Geometry: final body of the model. Coordinates: model frame, mm. Coordinates: 2 decimals unless noted, no trailing zeros. Loops run counter-clockwise (first coordinate to the right, second up) from the corner with the lowest first, then second, coordinate; pieces in that order, holes last. Notation, with made-up numbers: (-5.5, 32.25) - (12.5, 32.25) arc R33 cw to (12.5, 65.25) - close; hole circle Ø3 at (76, 13). An arc over 180 degrees is marked (long way). Put each result on its own line as item: value. Start each with the question number.
1) Material intervals for line 1 along Y through (x, z) = (257, 0.4); line 2 along Y through (x, z) = (217, -1.4); line 3 along X through (y, z) = (93, 0.8), sorted ascending. Write a range as from..to.
2) Section A-A on y = 108.5. Output: boundary loops of the cut face in (x, z), and give its area (3 significant figures).
3) Section D-D on x = 197. Output: boundary loops of the cut face in (y, z).
4) Section B-B on y = 123.5. Output: boundary loops of the cut face in (x, z), and give its area (3 significant figures).
5) Section C-C on y = 50. Output: boundary loops of the cut face in (x, z), and give its area (3 significant figures).
6) Contact query for flat-ended pins moving along their axis: pin 1 Ø0.9 at (y, z) = (124.5, -0.5) entering from +X; pin 2 Ø0.9 at (y, z) = (64.5, 0.5) entering from +X; pin 3 Ø0.9 at (x, z) = (262, 0.5) entering from +Y. Output: stop coordinate, or through.
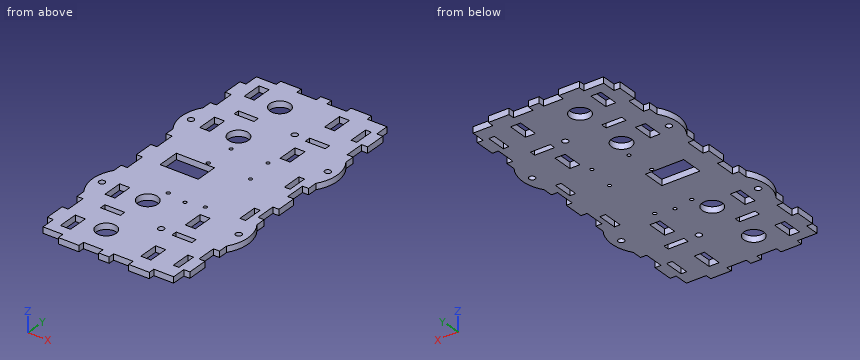
```python
from build123d import *

# Parameters (mm, degrees)
CROQUIS1_R                               = 1.5
CROQUIS1_R_2                             = 1.506117052
SALIENTE_EXTRUIR1_DEPTH                  = 1.5
CROQUIS3_W                               = 13
CROQUIS3_H                               = 10.999999999
CORTAR_EXTRUIR2_DEPTH                    = 10
TALADRO_DE_MARGEN_PARA_M1_61_D           = 1.7
TALADRO_DE_MARGEN_PARA_M1_61_CSINK_D     = 1.75
TALADRO_DE_MARGEN_PARA_M1_61_CSINK_ANGLE = 90
CROQUIS10_W                              = 5
CROQUIS10_H                              = 10
CORTAR_EXTRUIR3_DEPTH                    = 10
TALADRO_DE_MARGEN_PARA_M1_62_D           = 1.7
TALADRO_DE_MARGEN_PARA_M1_62_DEPTH       = 10
TALADRO_DE_MARGEN_PARA_M1_62_TIP         = 0.510731526
CROQUIS14_W                              = 2.8
CROQUIS14_H                              = 9.8
CORTAR_EXTRUIR4_DEPTH                    = 10
CROQUIS15_R                              = 5
CORTAR_EXTRUIR5_DEPTH                    = 10


with BuildPart() as part:
    # Croquis1 → Saliente-Extruir1 (new, symmetric)
    with BuildSketch(Plane.XY):
        with BuildLine():
            Line((205.355115241, 182.028523427), (195.480115242, 182.028523427))
            Line((195.480115242, 182.028523427), (195.480115242, 175.028523428))
            Line((195.480115242, 175.028523428), (192.480115242, 175.028523428))
            Line((192.480115242, 175.028523428), (192.480115242, 165.028523428))
            Line((192.480115242, 165.028523428), (195.480115242, 165.028523428))
            Line((195.480115242, 165.028523428), (195.480115242, 155.028523429))
            Line((195.480115242, 155.028523429), (192.480115242, 155.028523429))
            Line((192.480115242, 155.028523429), (192.480115242, 150.148106778))
            ThreePointArc((192.480115242, 150.148106778), (189.350724152, 139.96602343), (192.480115242, 129.783940083))
            Line((192.480115242, 129.783940083), (192.480115242, 125.153523431))
            Line((192.480115242, 125.153523431), (195.480115242, 125.153523431))
            Line((195.480115242, 125.153523431), (195.480115242, 114.903523432))
            Line((195.480115242, 114.903523432), (192.480115242, 114.903523432))
            Line((192.480115242, 114.903523432), (192.480115242, 105.153523433))
            Line((192.480115242, 105.153523433), (195.480115242, 105.153523433))
            Line((195.480115242, 105.153523433), (195.480115242, 94.903523434))
            Line((195.480115242, 94.903523434), (192.480115242, 94.903523434))
            Line((192.480115242, 94.903523434), (192.480115242, 90.023106782))
            ThreePointArc((192.480115242, 90.023106782), (189.350724152, 79.841023435), (192.480115242, 69.658940087))
            Line((192.480115242, 69.658940087), (192.480115242, 65.028523436))
            Line((192.480115242, 65.028523436), (195.480115242, 65.028523436))
            Line((195.480115242, 65.028523436), (195.480115242, 55.028523436))
            Line((195.480115242, 55.028523436), (192.480115242, 55.028523436))
            Line((192.480115242, 55.028523436), (192.480115242, 45.028523437))
            Line((192.480115242, 45.028523437), (195.480115242, 45.028523437))
            Line((195.480115242, 45.028523437), (195.480115242, 38.028637727))
            Line((195.480115242, 38.028637727), (205.355115241, 38.028637727))
            Line((205.355115241, 38.028637727), (205.355115241, 35.028637727))
            Line((205.355115241, 35.028637727), (215.605115241, 35.028637727))
            Line((215.605115241, 35.028637727), (215.605115241, 38.028620144))
            Line((215.605115241, 38.028620144), (225.355044383, 38.028620144))
            Line((225.355044383, 38.028620144), (225.355044383, 35.028598165))
            Line((225.355044383, 35.028598165), (230.605044383, 35.028598165))
            Line((230.605044383, 35.028598165), (230.605044383, 38.028598165))
            Line((230.605044383, 38.028598165), (240.354973525, 38.028598165))
            Line((240.354973525, 38.028598165), (240.354973525, 35.028589374))
            Line((240.354973525, 35.028589374), (250.604973524, 35.028589374))
            Line((250.604973524, 35.028589374), (250.604973524, 38.028580582))
            Line((250.604973524, 38.028580582), (260.479973524, 38.028580582))
            Line((260.479973524, 38.028580582), (260.479973524, 44.903580582))
            Line((260.479973524, 44.903580582), (263.479973523, 44.903580582))
            Line((263.479973523, 44.903580582), (263.479973523, 55.153580581))
            Line((263.479973523, 55.153580581), (260.479973524, 55.153580581))
            Line((260.479973524, 55.153580581), (260.479973524, 64.90358058))
            Line((260.479973524, 64.90358058), (263.479973523, 64.90358058))
            Line((263.479973523, 64.90358058), (263.479973523, 69.783997232))
            ThreePointArc((263.479973523, 69.783997232), (266.609364614, 79.966080579), (263.479973523, 90.148163927))
            Line((263.479973523, 90.148163927), (263.479973523, 95.028580578))
            Line((263.479973523, 95.028580578), (260.479973524, 95.028580578))
            Line((260.479973524, 95.028580578), (260.479973524, 105.028580577))
            Line((260.479973524, 105.028580577), (263.479973523, 105.028580577))
            Line((263.479973523, 105.028580577), (263.479973523, 115.028580577))
            Line((263.479973523, 115.028580577), (260.479973524, 115.028580577))
            Line((260.479973524, 115.028580577), (260.479973524, 125.028580576))
            Line((260.479973524, 125.028580576), (263.479973523, 125.028580576))
            Line((263.479973523, 125.028580576), (263.479973523, 129.908997227))
            ThreePointArc((263.479973523, 129.908997227), (266.609364614, 140.091080575), (263.479973523, 150.273163922))
            Line((263.479973523, 150.273163922), (263.479973523, 155.153580574))
            Line((263.479973523, 155.153580574), (260.479973524, 155.153580574))
            Line((260.479973524, 155.153580574), (260.479973524, 164.903580573))
            Line((260.479973524, 164.903580573), (263.479973523, 164.903580573))
            Line((263.479973523, 164.903580573), (263.479973523, 175.153580572))
            Line((263.479973523, 175.153580572), (260.479973524, 175.153580572))
            Line((260.479973524, 175.153580572), (260.479973524, 182.028580572))
            Line((260.479973524, 182.028580572), (250.604973524, 182.028580572))
            Line((250.604973524, 182.028580572), (250.604973524, 185.02857178))
            Line((250.604973524, 185.02857178), (240.354973525, 185.02857178))
            Line((240.354973525, 185.02857178), (240.354973525, 182.028562989))
            Line((240.354973525, 182.028562989), (230.605044383, 182.028562989))
            Line((230.605044383, 182.028562989), (230.605044383, 185.028562989))
            Line((230.605044383, 185.028562989), (225.355044383, 185.028562989))
            Line((225.355044383, 185.028562989), (225.355044383, 182.02854101))
            Line((225.355044383, 182.02854101), (215.605115241, 182.02854101))
            Line((215.605115241, 182.02854101), (215.605115241, 185.028523427))
            Line((215.605115241, 185.028523427), (205.355115241, 185.028523427))
            Line((205.355115241, 185.028523427), (205.355115241, 182.028523427))
        make_face()
        Polygon((215.180079812, 63.578494864), (210.095175212, 63.578494864), (205.280079813, 63.578494864), (205.280079813, 65.17614563), (205.280079813, 66.478494863), (210.095175212, 66.478494863), (215.180079812, 66.478494863), (215.180079812, 65.17614563), align=None, mode=Mode.SUBTRACT)
        with Locations((193.980115242, 79.841023435)):
            Circle(CROQUIS1_R, mode=Mode.SUBTRACT)
        Polygon((204.687627513, 115.528523432), (207.487627511, 115.528523432), (210.687627512, 115.528523432), (210.687627512, 109.828523436), (210.687627512, 104.528523433), (207.487627511, 104.528523433), (204.687627513, 104.528523433), (204.687627513, 110.228523436), align=None, mode=Mode.SUBTRACT)
        with Locations((234.380026668, 65.028523436)):
            Circle(CROQUIS1_R_2, mode=Mode.SUBTRACT)
        Polygon((250.680008953, 63.578523436), (245.595104353, 63.578523436), (240.780008954, 63.578523436), (240.780008954, 65.176174202), (240.780008954, 66.478523436), (245.595104353, 66.478523436), (250.680008953, 66.478523436), (250.680008953, 65.176174202), align=None, mode=Mode.SUBTRACT)
        with Locations((261.979973524, 79.966080579)):
            Circle(CROQUIS1_R, mode=Mode.SUBTRACT)
        with Locations((193.980115242, 139.96602343)):
            Circle(CROQUIS1_R, mode=Mode.SUBTRACT)
        Polygon((215.180079812, 153.675173656), (210.095175212, 153.675173656), (205.280079813, 153.675173656), (205.280079813, 155.272824422), (205.280079813, 156.575173656), (210.095175212, 156.575173656), (215.180079812, 156.575173656), (215.180079812, 155.272824422), align=None, mode=Mode.SUBTRACT)
        with Locations((261.979973524, 140.091080575)):
            Circle(CROQUIS1_R, mode=Mode.SUBTRACT)
        with Locations((234.380026668, 155.125202228)):
            Circle(CROQUIS1_R, mode=Mode.SUBTRACT)
        Polygon((250.680008953, 153.675202228), (245.864913553, 153.675202228), (240.780008954, 153.675202228), (240.780008954, 155.272852994), (240.780008954, 156.575202228), (245.864913553, 156.575202228), (250.680008953, 156.575202228), (250.680008953, 155.272852994), align=None, mode=Mode.SUBTRACT)
    extrude(amount=SALIENTE_EXTRUIR1_DEPTH, both=True)

    # Croquis3 → Cortar-Extruir2 (cut)
    with BuildSketch(Plane(origin=(0, 0, -1.5), x_dir=(-1, 0, 0), z_dir=(0, 0, -1))):
        with Locations((-217.187627512, 110.028523433)):
            Rectangle(CROQUIS3_W, CROQUIS3_H)
    extrude(amount=-CORTAR_EXTRUIR2_DEPTH, mode=Mode.SUBTRACT)

    # Taladro de margen para M1.61 (through all)
    with Locations(Plane(origin=(0, 0, -1.5), x_dir=(-1, 0, 0), z_dir=(0, 0, -1))):
        with Locations((-238.760115242, 131.208523432), (-220.340115242, 131.208523432), (-220.340115242, 88.848637722), (-238.760115242, 88.848637722)):
            CounterSinkHole(TALADRO_DE_MARGEN_PARA_M1_61_D / 2, TALADRO_DE_MARGEN_PARA_M1_61_CSINK_D / 2, counter_sink_angle=TALADRO_DE_MARGEN_PARA_M1_61_CSINK_ANGLE)

    # Croquis10 → Cortar-Extruir3 (cut)
    with BuildSketch(Plane(origin=(0, 0, -1.5), x_dir=(-1, 0, 0), z_dir=(0, 0, -1))):
        with Locations((-202.980115242, 142.028580577)):
            Rectangle(CROQUIS10_W, CROQUIS10_H)
        with Locations((-202.980115242, 172.028580577)):
            Rectangle(CROQUIS10_W, CROQUIS10_H)
        with Locations((-202.980115242, 78.028580577)):
            Rectangle(CROQUIS10_W, CROQUIS10_H)
        with Locations((-202.980115242, 48.028580577)):
            Rectangle(CROQUIS10_W, CROQUIS10_H)
        with Locations((-242.980115242, 48.028580577)):
            Rectangle(CROQUIS10_W, CROQUIS10_H)
        with Locations((-242.980115242, 78.028580577)):
            Rectangle(CROQUIS10_W, CROQUIS10_H)
        with Locations((-242.980115242, 172.028580577)):
            Rectangle(CROQUIS10_W, CROQUIS10_H)
        with Locations((-242.980115242, 142.028580577)):
            Rectangle(CROQUIS10_W, CROQUIS10_H)
    extrude(amount=-CORTAR_EXTRUIR3_DEPTH, mode=Mode.SUBTRACT)

    # Taladro de margen para M1.62
    with Locations(Plane(origin=(0, 0, -1.5), x_dir=(-1, 0, 0), z_dir=(0, 0, -1))):
        with Locations((-240.479973524, 117.029100767), (-219.479973524, 117.029100767), (-229.979973524, 87.029100767), (-170.093156085, 124.870857212)):
            Hole(TALADRO_DE_MARGEN_PARA_M1_62_D / 2, depth=TALADRO_DE_MARGEN_PARA_M1_62_DEPTH)
            with Locations((0, 0, -(TALADRO_DE_MARGEN_PARA_M1_62_DEPTH + TALADRO_DE_MARGEN_PARA_M1_62_TIP / 2))):  # 118° drill point
                Cone(0, TALADRO_DE_MARGEN_PARA_M1_62_D / 2, TALADRO_DE_MARGEN_PARA_M1_62_TIP, mode=Mode.SUBTRACT)

    # Croquis14 → Cortar-Extruir4 (cut)
    with BuildSketch(Plane(origin=(0, 0, -1.5), x_dir=(-1, 0, 0), z_dir=(0, 0, -1))):
        with Locations((-256.479973523, 170.028574939)):
            Rectangle(CROQUIS14_W, CROQUIS14_H)
        with Locations((-256.479973523, 50.028586215)):
            Rectangle(CROQUIS14_W, CROQUIS14_H)
        with Locations((-256.479973523, 95.028580577)):
            Rectangle(CROQUIS14_W, CROQUIS14_H)
        with Locations((-256.479973523, 125.028580577)):
            Rectangle(CROQUIS14_W, CROQUIS14_H)
    extrude(amount=-CORTAR_EXTRUIR4_DEPTH, mode=Mode.SUBTRACT)

    # Croquis15 → Cortar-Extruir5 (cut)
    with BuildSketch(Plane(origin=(0, 0, -1.5), x_dir=(-1, 0, 0), z_dir=(0, 0, -1))):
        with Locations((-217.080079819, 51.410663554)):
            Circle(CROQUIS15_R)
        with Locations((-217.080079819, 79.410663554)):
            Circle(CROQUIS15_R)
        with Locations(Location((-217.080079819, 140.6464976, 0), (0, 0, 180))):
            Circle(CROQUIS15_R)
        with Locations(Location((-217.080079819, 168.6464976, 0), (0, 0, 180))):
            Circle(CROQUIS15_R)
    extrude(amount=-CORTAR_EXTRUIR5_DEPTH, mode=Mode.SUBTRACT)


solid = part.part
```
Answer block:
1. line 1: y = 38.03..45.13, 54.93..90.13, 99.93..120.13, 129.93..165.13, 174.93..182.03
1. line 2: y = 38.03..46.41, 56.41..74.41, 84.41..104.53, 115.53..135.65, 145.65..163.65, 173.65..182.03
1. line 3: x = 192.48..255.08, 257.88..263.48
2. outline: (192.48, -1.5) - (204.69, -1.5) - (204.69, 1.5) - (192.48, 1.5) - close; (223.69, -1.5) - (263.48, -1.5) - (263.48, 1.5) - (223.69, 1.5) - close
2. area: 156 mm²
3. outline: (38.03, -1.5) - (182.03, -1.5) - (182.03, 1.5) - (38.03, 1.5) - close
4. outline: (195.48, -1.5) - (255.08, -1.5) - (255.08, 1.5) - (195.48, 1.5) - close; (257.88, -1.5) - (260.48, -1.5) - (260.48, 1.5) - (257.88, 1.5) - close
4. area: 187 mm²
5. outline: (192.48, -1.5) - (200.48, -1.5) - (200.48, 1.5) - (192.48, 1.5) - close; (205.48, -1.5) - (212.28, -1.5) - (212.28, 1.5) - (205.48, 1.5) - close; (221.88, -1.5) - (240.48, -1.5) - (240.48, 1.5) - (221.88, 1.5) - close; (245.48, -1.5) - (255.08, -1.5) - (255.08, 1.5) - (245.48, 1.5) - close; (257.88, -1.5) - (263.48, -1.5) - (263.48, 1.5) - (257.88, 1.5) - close
5. area: 146 mm²
6. pin 1: stops at x = 260.48
6. pin 2: stops at x = 263.48
6. pin 3: stops at y = 175.15
